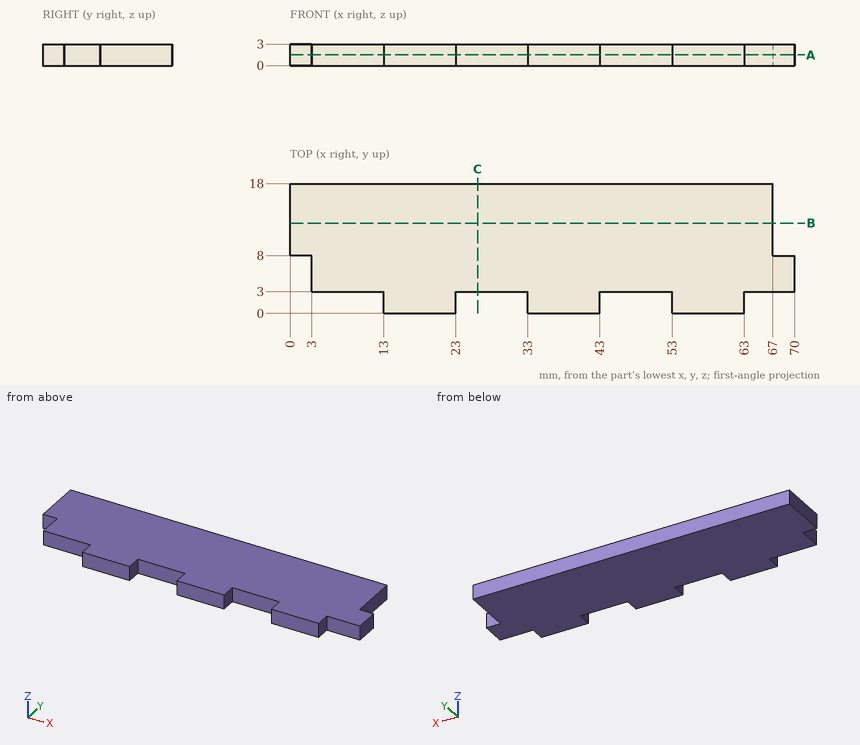
Input: dimensioned drawing with shaded views. Units: mm. Origin: part minimum x, y, z. Give positions to 0.01 mm unless a question says otherwise; leave off trailing zeros. Write each loop counter-clockwise with the first axis right and the second up, starting at its lowest first coordinate (ties: lowest second). Pieces come first, ordered by that corner, then holes. Notation, with made-up numbers: (53, 2.25) - (106, 2.25) arc R8 cw to (106, 8.25) - close; hole circle Ø2 at (5, 14.5). An arc over 180 degrees is marked (long way). One line per item, written item: value. Start each with the question number.
Q1. Material intervals for probe 1 along X at (y, z) = (2, 2.25); probe 2 along X at (y, z) = (10, 2.85); probe 3 along Y at (x, z) = (50, 1.95), sorted ascending. Write a range as from..to.
Q2. Section query A-A, the plane z = 1.5. Return the cut outline in (x, y), then the cut area to 4 significant figures.
Q3. Section query B-B, the plane y = 12.5. Return the cut outline in (x, z).
Q4. Section query C-C, the plane x = 26. Return the cut outline in (y, z).
Q5. First-contact query: pin 1 Ø0.9 at (x, z) = (65.5, 1.5) entering from -Y; pin 2 Ø1.5 at (y, z) = (2, 1) entering from +X; pin 3 Ø0.9 at (y, z) = (1.5, 1) entering from -X. Flat tips, straight axial feed; report the tip coordinate or a pass-through.
Answer:
1. probe 1: x = 13..23, 33..43, 53..63
1. probe 2: x = 0..67
1. probe 3: y = 3..18
2. outline: (0, 8) - (3, 8) - (3, 3) - (13, 3) - (13, 0) - (23, 0) - (23, 3) - (33, 3) - (33, 0) - (43, 0) - (43, 3) - (53, 3) - (53, 0) - (63, 0) - (63, 3) - (70, 3) - (70, 8) - (67, 8) - (67, 18) - (0, 18) - close
2. area: 1,095 mm2
3. outline: (0, 0) - (67, 0) - (67, 3) - (0, 3) - close
4. outline: (3, 0) - (18, 0) - (18, 3) - (3, 3) - close
5. pin 1: stops at y = 3
5. pin 2: stops at x = 63
5. pin 3: stops at x = 13
